from build123d import *

# Parameters (mm, degrees)
SKETCH1_R           = 9.4
BOSS_EXTRUDE1_DEPTH = 5.8
SKETCH2_R           = 7.95
CUT_EXTRUDE1_DEPTH  = 3.2
SKETCH3_R           = 1
BOSS_EXTRUDE2_DEPTH = 1.5875
SKETCH4_R           = 3.7
BOSS_EXTRUDE3_DEPTH = 3
SKETCH5_R           = 1.4
CUT_EXTRUDE2_DEPTH  = 41.270506735
CHAMFER2_SIZE       = 1.477787454
CHAMFER2_SIZE_2     = 1.7


with BuildPart() as part:
    # Sketch1 → Boss-Extrude1 (new body)
    with BuildSketch(Plane.XY):
        with Locations((-29.082250471, -1.703826149)):
            Circle(SKETCH1_R)
    extrude(amount=BOSS_EXTRUDE1_DEPTH)

    # Sketch2 → Cut-Extrude1 (cut)
    with BuildSketch(Plane(origin=(0, 0, 0), x_dir=(-1, 0, 0), z_dir=(0, 0, -1))):
        with Locations((29.082250471, -1.703826149)):
            Circle(SKETCH2_R)
    extrude(amount=-CUT_EXTRUDE1_DEPTH, mode=Mode.SUBTRACT)

    # Sketch3 → Boss-Extrude2 (add)
    with BuildSketch(Plane(origin=(0, 0, 3.2), x_dir=(-1, 0, 0), z_dir=(0, 0, -1))):
        with Locations((29.082250471, -1.703826149)):
            Circle(SKETCH3_R)
    extrude(amount=BOSS_EXTRUDE2_DEPTH)

    # Sketch4 → Boss-Extrude3 (add)
    with BuildSketch(Plane(origin=(0, 0, 1.6125), x_dir=(-1, 0, 0), z_dir=(0, 0, -1))):
        with Locations((29.082250471, -1.703826149)):
            Circle(SKETCH4_R)
    extrude(amount=-BOSS_EXTRUDE3_DEPTH)

    # Sketch5 → Cut-Extrude2 (cut, through all)
    with BuildSketch(Plane(origin=(0, 0, 1.6125), x_dir=(-1, 0, 0), z_dir=(0, 0, -1))):
        with Locations((29.082250471, -1.703826149)):
            Circle(SKETCH5_R)
    extrude(amount=-CUT_EXTRUDE2_DEPTH, mode=Mode.SUBTRACT)

    # Chamfer2
    # the kernel refuses this chamfer: 1.7, 1.477787454 mm, written as the material it takes off along each edge
    with BuildSketch(Plane(origin=(-29.082250471, -1.703826149, 1.6125), x_dir=(-1, 0, 0), z_dir=(0, -1, 0))) as chamfer2_piece_1_section:
        Polygon((3.7 - CHAMFER2_SIZE, 0), (3.7, -CHAMFER2_SIZE_2), (3.7, 0), align=None)
    chamfer2_piece_1 = revolve(axis=Axis((-29.082250471, -1.703826149, 1.6125), (0, 0, -1)), mode=Mode.PRIVATE)
    chamfer2_piece_1 = split(chamfer2_piece_1, bisect_by=Plane(origin=(-26.169502039, -1.703826149, 3.2), z_dir=(0, 0, -1)), keep=Keep.TOP, mode=Mode.PRIVATE)
    add(chamfer2_piece_1, mode=Mode.SUBTRACT)


solid = part.part
The model under review builds one solid part; all positions refer to its coordinate system, in mm. A direction names the side the tool comes from. Round coordinates to 2 decimals unless told otherwise and drop trailing zeros. Write each loop counter-clockwise with the first axis right and the second up, starting at its lowest first coordinate (ties: lowest second). Pieces come first, ordered by that corner, then holes. Notation, with made-up numbers: (76.25, 28) -> (80.25, 28) arc R22 ccw to (80.25, 47) -> close; hole circle Ø1 at (20, 65). An arc over 180 degrees is marked (long way). Answer as a JSON object with one key per item and string values.
1. We need section B-B on x = -24. State the section outline as (y, z) points, and give its area (3 significant figures).
Results found:
{"outline": "(-9.61, 0) -> (-7.82, 0) -> (-7.82, 3.2) -> (4.41, 3.2) -> (4.41, 0) -> (6.2, 0) -> (6.2, 5.8) -> (-9.61, 5.8) -> close", "area": "52.6 mm^2"}
2. The part is to be moulded in two halves that separate along Y. For faces 1 (the face through (-20.116, 1.12, 2.859)), 2 (the face through (-31, -2, 1.612)), 3 (the face through (-33, -3, 3.2)), 4 (the face through (-27, -2, 5.8)), say which applies: pulls with the +Y half, pulls with the -Y half, needs draft (parallel to the pull), parting line crosses it, or undercut.
Results found:
{"face 1": "parting line crosses it", "face 2": "undercut", "face 3": "undercut", "face 4": "needs draft"}
3. We need section C-C on y = -6.25. State the section outline as (x, z) points, and give its area (3 significant figures).
Results found:
{"outline": "(-37.31, 0) -> (-35.6, 0) -> (-35.6, 3.2) -> (-22.56, 3.2) -> (-22.56, 0) -> (-20.85, 0) -> (-20.85, 5.8) -> (-37.31, 5.8) -> close", "area": "53.7 mm^2"}
4. Machinability: for faces 5 (the face through (-27.684, -1.642, 3.677)), 6 (the face through (-27.359, -9.465, 1.578)), which of the approach directions +Z, -Z, +X, -X, +Y, -Y give a long, thin tool a straight path to every point of the face, cutting with its end or side? Answer none if there is none.
Results found:
{"face 5": "+Z, -Z", "face 6": "-Z"}
5. We need section D-D on z = 0.75. State the section outline as (x, y) points, and give its area (3 significant figures).
Results found:
{"outline": "circle Ø18.8 at (-29.08, -1.7); hole circle Ø15.9 at (-29.08, -1.7)", "area": "79.0 mm^2"}
6. To check wall thickness, follow line 1 along X through (y, z) = (-1.75, 5.2); line 2 along X through (y, z) = (-2.5, 2.2); line 3 along Y through (x, z) = (-27.25, 2.35). State the ranges of each line that lie inside material, in increasing order.
Results found:
{"line 1": "x = -38.48 to -30.48, -27.68 to -19.68", "line 2": "x = -38.45 to -36.99, -31.7 to -30.23, -27.93 to -26.47, -21.17 to -19.72", "line 3": "y = -10.92 to -9.44, -3.9 to 0.5, 6.03 to 7.52"}
7. We need section A-A on z = 2.95. State the section outline as (x, y) points.
Results found:
{"outline": "circle Ø18.8 at (-29.08, -1.7); circle Ø6.77 at (-29.08, -1.7); hole circle Ø15.9 at (-29.08, -1.7); hole circle Ø2.8 at (-29.08, -1.7)"}
8. Clearance check with flat-ended pins moving along their axes: pin 1 (3 mm diameter, centred on x = -34, z = 1.5, fed in from +Y); pin 2 (1 mm diameter, centred on y = -6.5, z = 2.5, fed in from +X); pin 3 (1.5 mm diameter, centred on x = -22.5, y = 1, fed in from -Z). State where each tip first meets the part, or that it passes through.
Results found:
{"pin 1": "stops at y = 7.05", "pin 2": "stops at x = -20.72", "pin 3": "stops at z = 3.2"}
